Autodesk Inventor part; units mm, degrees
ref_plane "YZ Plane" through (0, 0, 0) normal (1, 0, 0) x (0, 1, 0)
ref_plane "XZ Plane" through (0, 0, 0) normal (0, 1, 0) x (-1, 0, 0)
ref_plane "XY Plane" through (0, 0, 0) normal (0, 0, 1) x (1, 0, 0)
sketch "Sketch1" plane through (0, 0, 0) normal (0, 1, 0) x (-1, 0, 0)
  line L0 (0, 0) -> (38, 0)
  line L1 (38, 0) -> (38, -38)
  line L2 (38, -38) -> (0, -38)
  line L3 (0, -38) -> (0, 0)
  line L4 (19, 0) -> (19, -38)
  line L5 (38, -19) -> (0, -19)
  circle A0 centre (19, -19) radius 8
  line L6 (0, -19) -> (0, -5)
  line L7 (38, -19) -> (38, -5)
  line L8 (38, -19) -> (38, -33)
  line L9 (0, -19) -> (0, -33)
  line L10 (0, -33) -> (38, -33)
  line L11 (38, -5) -> (0, -5)
  line L12 (19, -5) -> (5, -5)
  line L13 (19, -33) -> (33, -33)
  line L14 (33, -33) -> (33, -5)
  line L15 (5, -5) -> (5, -33)
  circle A1 centre (5, -5) radius 1
  circle A2 centre (5, -33) radius 1
  circle A3 centre (33, -33) radius 1
  circle A4 centre (33, -5) radius 1
  dimension "d0" = 38
  dimension "d1" = 38
  dimension "d2" = 16
  dimension "d3" = 14
  dimension "d4" = 14
  dimension "d5" = 14
  dimension "d6" = 14
  dimension "d7" = 14
  dimension "d8" = 14
  dimension "d9" = 28
  dimension "d10" = 28
  dimension "d11" = 2
  dimension "d12" = 2
  dimension "d13" = 2
  dimension "d14" = 2
extrude "Extrusion1" add sketch "Sketch1" along normal blind 1.5 contours L0 L4 L11 A1 L3 | L0 L1 L11 A4 L4 | L11 A1 L15 L5 L3 | L11 A4 L14 L5 A0 L4 | L4 A0 L5 L15 A1 L11 | L5 L15 A2 L10 L3 | L1 L5 L14 A4 L11 | L10 A2 L4 L2 L3 | L5 A0 L4 L10 A2 L15 | L1 L10 A3 L14 L5 | L5 L14 A3 L10 L4 A0 | L1 L2 L4 L10 A3
sketch "Sketch2" plane through (0, 0, 0) normal (0, -1, 0) x (1, 0, 0)
  circle A0 centre (-19, -19) radius 8
  circle A1 centre (-19, -19) radius 8
  point P0 (0, 0)
extrude "Extrusion2" add sketch "Sketch2" against normal blind 22
sketch "Sketch4" plane through (0, 0, 0) normal (0, -1, 0) x (1, 0, 0)
  line L0 (0, 0) -> (0, -38)
  line L1 (0, -19) -> (-38, -19)
  line L2 (-38, -38) -> (-38, 0)
  line L3 (0, -38) -> (-38, -38)
  line L4 (-19, -38) -> (-19, 0)
  line L5 (-19, -19) -> (-19, -1.75)
  line L6 (-19, -1.75) -> (-1.75, -1.75)
  line L7 (-19, -19) -> (-36.25, -19)
  line L8 (-36.25, -19) -> (-36.25, -36.25)
  circle A0 centre (-1.75, -1.75) radius 1
  circle A1 centre (-36.25, -36.25) radius 1
  circle A2 centre (-1.75, -36.25) radius 1
  circle A3 centre (-36.25, -1.75) radius 1
  dimension "d24" = 17.25
  dimension "d25" = 17.25
  dimension "d26" = 17.25
  dimension "d27" = 17.25
  dimension "d28" = 2
  dimension "d29" = 2
extrude "Extrusion4" cut sketch "Sketch4" against normal blind 10 contours A0 | A1 | A2 | A3
properties part number "camera_v1"
Input: part model. Units: mm. Frame: model coordinates. A direction names the side the tool comes from. Coordinates: 2 decimals unless noted, no trailing zeros. Order: outer loops, then holes, each group sorted by start corner. A loop starts at its lowest first (then second) coordinate and runs counter-clockwise, first axis right, second up. Notation, with made-up numbers: (-16, 62) - (13, 62) arc R20 ccw to (13, 75) - close; hole circle Ø2 at (22, 13). An arc over 180 degrees is marked (long way). Return JSON: item names as keys, results as strings.
Q1. Cut plane D-D (y = 20). Return loops of the section in (x, z), then the cut area to 3 significant figures.
The answers:
{"outline": "circle Ø16 at (-19, -19)", "area": "201 mm2"}
Q2. First-contact query: pin 1 (2 mm diameter, centred on x = -5, z = -21, fed in from +Y); pin 2 (10 mm diameter, centred on x = -26, y = 18, fed in from -Z); pin 3 (1.8 mm diameter, centred on x = -5, z = -5, fed in from -Y); pin 4 (8 mm diameter, centred on x = -26, y = 19, fed in from -Z). Flat tips, straight axial feed; report the tip coordinate or a pass-through.
The answers:
{"pin 1": "stops at y = 1.5", "pin 2": "stops at z = -26.75", "pin 3": "passes through", "pin 4": "stops at z = -26.42"}
Q3. Cut plane B-B (x = -1.75). Return loops of the section in (y, z).
The answers:
{"outline": "(0, -38) - (1.5, -38) - (1.5, -37.25) - (0, -37.25) - close; (0, -35.25) - (1.5, -35.25) - (1.5, -2.75) - (0, -2.75) - close; (0, -0.75) - (1.5, -0.75) - (1.5, 0) - (0, 0) - close"}
Q4. Ray query, probe 1 along Z at (x, y) = (-5, 0.8); probe 2 along Z at (x, y) = (-1.75, 0.3). Return the intervals inside material, ascending.
The answers:
{"probe 1": "z = -38 to -34, -32 to -6, -4 to 0", "probe 2": "z = -38 to -37.25, -35.25 to -2.75, -0.75 to 0"}
Q5. Cut plane A-A (z = -33). Return loops of the section in (x, y), then the cut area to 3 significant figures.
The answers:
{"outline": "(-38, 0) - (-34, 0) - (-34, 1.5) - (-38, 1.5) - close; (-32, 0) - (-6, 0) - (-6, 1.5) - (-32, 1.5) - close; (-4, 0) - (0, 0) - (0, 1.5) - (-4, 1.5) - close", "area": "51.0 mm2"}
Q6. Cut plane C-C (z = -19). Return loops of the section in (x, y), then the cut area to 3 significant figures.
The answers:
{"outline": "(-38, 0) - (0, 0) - (0, 1.5) - (-11, 1.5) - (-11, 22) - (-27, 22) - (-27, 1.5) - (-38, 1.5) - close", "area": "385 mm2"}
Q7. Access query for faces 1 (the flat face through (-18.7, 1.5, -27.2)), 2 (the cylindrical face through (-1.88, 0.74, -35.26)). Directions: +Z, -Z, +X, -X, +Y, -Y. A direction counts if a zero-diameter tool reaches every point of the face in a straight line with its end or side. Return the directions, or none.
The answers:
{"face 1": "+Y", "face 2": "+Y, -Y"}
